Source: CAD feature listing. Evaluate the final solid. Frame: model axes, mm. Coordinates: 2 decimals unless noted, no trailing zeros. Answer as CSV lines item,"result".
from build123d import *

# Parameters (mm, degrees)
MAIN_PROFILE_SKETCH_W   = 143.5
MAIN_PROFILE_SKETCH_H   = 580
MAIN_PROFILE_SKETCH_R   = 1.7
MAIN_PROFILE_SKETCH_R_2 = 11.2
MAIN_EXTRUSION_DEPTH    = 1.5


with BuildPart() as part:
    # Main Profile Sketch → Main Extrusion (new body)
    with BuildSketch(Plane.XY.offset(111.5)):
        with Locations((-213.25, 0)):
            Rectangle(MAIN_PROFILE_SKETCH_W, MAIN_PROFILE_SKETCH_H)
        with Locations((-255, -285)):
            Circle(MAIN_PROFILE_SKETCH_R, mode=Mode.SUBTRACT)
        with Locations((-146.5, -250)):
            Circle(MAIN_PROFILE_SKETCH_R, mode=Mode.SUBTRACT)
        with Locations((-250, 0)):
            Circle(MAIN_PROFILE_SKETCH_R_2, mode=Mode.SUBTRACT)
        with Locations((-255, 285)):
            Circle(MAIN_PROFILE_SKETCH_R, mode=Mode.SUBTRACT)
        with Locations((-146.5, 0)):
            Circle(MAIN_PROFILE_SKETCH_R, mode=Mode.SUBTRACT)
        with Locations((-146.5, 250)):
            Circle(MAIN_PROFILE_SKETCH_R, mode=Mode.SUBTRACT)
    extrude(amount=-MAIN_EXTRUSION_DEPTH)


solid = part.part
(1) Draft query along Y for faces 1 (the flat face through (-214, 4, 111.5)), 2 (the cylindrical face through (-261.19, 0.49, 110.76)). Return one class per face: released by +Y, released by -Y, zero draft, split by the parting line, or undercut.
Computed values:
face 1,"zero draft"
face 2,"undercut"
(2) Material intervals for L1, parallel to Y at x = -146.5, z = 111; L2, parallel to Y at x = -253.5, z = 111.15; L3, parallel to X at y = -250, z = 110.7, sorted ascending. Write a range as [from, to].
Computed values:
L1,"[-290, -251.7], [-248.3, -1.7], [1.7, 248.3], [251.7, 290]"
L2,"[-290, -285.8], [-284.2, -10.64], [10.64, 284.2], [285.8, 290]"
L3,"[-285, -148.2], [-144.8, -141.5]"
(3) Pin query (flat end, axial travel): pin 1 Ø13.5 at (x, y) = (-250, 0) entering from -Z; pin 2 Ø4 at (x, y) = (-146.5, 0) entering from -Z. Return the tip coordinate at first contact, or that it passes through.
Computed values:
pin 1,"through"
pin 2,"z = 110"
